```python
from build123d import *

# Parameters (mm, degrees)
BOSS_EXTRUDE1_DEPTH = 11
SHELL2_T            = -1.75
SKETCH5_W           = 10
SKETCH5_H           = 10.669048105
BOSS_EXTRUDE2_DEPTH = 9.25
HOLE4_D             = 4
HOLE4_DEPTH         = 13
HOLE4_CBORE_D       = 8
HOLE4_CBORE_DEPTH   = 5.5
HOLE4_TIP           = 1.201721238


with BuildPart() as part:
    # Sketch1 → Boss-Extrude1 (new body)
    with BuildSketch(Plane(origin=(0, 0, 0), x_dir=(1, 0, 0), z_dir=(0, 1, 0))):
        with BuildLine():
            Line((-12, -7.169048105), (-12, 13))
            Line((-12, 13), (12, 13))
            Line((12, 13), (12, -7.169048105))
            ThreePointArc((12, -7.169048105), (11.350863635, -11.062362212), (9.473684211, -14.534461025))
            ThreePointArc((9.473684211, -14.534461025), (7.719611593, -14.754072618), (7.5, -13))
            ThreePointArc((7.5, -13), (0, 2.330951895), (-7.5, -13))
            ThreePointArc((-7.5, -13), (-7.719611593, -14.754072618), (-9.473684211, -14.534461025))
            ThreePointArc((-9.473684211, -14.534461025), (-11.350863635, -11.062362212), (-12, -7.169048105))
        make_face()
    extrude(amount=BOSS_EXTRUDE1_DEPTH)

    # Shell2
    shell2_openings = [part.faces().sort_by_distance(p)[0] for p in [
        (0, 11, -3.682863913),
    ]]
    offset(amount=SHELL2_T, openings=shell2_openings, kind=Kind.INTERSECTION)

    # Sketch5 → Boss-Extrude2 (add)
    with BuildSketch(Plane(origin=(0, 11, 0), x_dir=(1, 0, 0), z_dir=(0, 1, 0))):
        with Locations((0, 7.665475948)):
            Rectangle(SKETCH5_W, SKETCH5_H)
    extrude(amount=-BOSS_EXTRUDE2_DEPTH)

    # Hole4
    with Locations(Plane.XY):
        with Locations((0, 5.5)):
            CounterBoreHole(HOLE4_D / 2, HOLE4_CBORE_D / 2, HOLE4_CBORE_DEPTH, depth=HOLE4_DEPTH)
            with Locations((0, 0, -(HOLE4_DEPTH + HOLE4_TIP / 2))):  # 118° drill point
                Cone(0, HOLE4_D / 2, HOLE4_TIP, mode=Mode.SUBTRACT)


solid = part.part
```
Build history of the part. All positions in model axes, mm. A direction names the side the tool comes from. Round coordinates to 2 decimals unless told otherwise and drop trailing zeros. Write each loop counter-clockwise with the first axis right and the second up, starting at its lowest first coordinate (ties: lowest second). Pieces come first, ordered by that corner, then holes.
1) Band-saw the part on B-B, the plane z = -6. List the corners of the cut face in (x, y).
2) Mould opens along Y. For faces 3 (the cylindrical face through (-7.7, 5.42, 14.74)), 4 (the cylindrical face through (2.15, 8.873, -3.446)), 5 (the flat face through (-8, 1.75, -6)) say: +Y half, -Y half, draft (parallel to the pull), parting line (faces both ways), or undercut.
3) 3-axis set-ups, long thin cutter, end or side, ignore diameter. For faces 1 (the flat face through (0, 3, -13)), 2 (the flat face through (5, 6, -7)): which of +Z, -Z, +X, -X, +Y, -Y reach the whole face in a straight line?
4) Band-saw the part on A-A, the plane y = 5.5. List the corners of the cut face in (x, z), and give its area (3 significant figures).
5) Pin check, flat tips, straight feed: pin 1 (4 mm diameter, centred on x = 6.5, y = 8.5, fed in from +Z); pin 2 (4 mm diameter, centred on x = -7.5, z = -5.5, fed in from +Y); pin 3 (2 mm diameter, centred on x = -0.5, y = 7.5, fed in from +Z); pin 4 (5 mm diameter, centred on x = 2.5, y = 1, fed in from +Z). Stop position of each tip, or through.
6) Band-saw the part on C-C, the plane x = 0. List the corners of the cut face in (y, z).
7) Band-saw the part on D-D, the plane z = 6.25. List the corners of the cut face in (x, y), and give its area (3 significant figures).
8) Drill centre lines: probe 1 along X at (y, z) = (5.5, -4.55); probe 2 along X at (y, z) = (9.75, 7); probe 3 along Y at (x, z) = (0, -8). Where is each one in solid material? Low to high.
Ans:
1. outline: (-12, 0) - (12, 0) - (12, 11) - (10.25, 11) - (10.25, 1.75) - (5, 1.75) - (5, 11) - (-5, 11) - (-5, 1.75) - (-10.25, 1.75) - (-10.25, 11) - (-12, 11) - close; hole circle Ø4 at (0, 5.5)
2. face 3: draft
2. face 4: undercut
2. face 5: +Y half
3. face 1: -Z, +X, -X, +Y, -Y
3. face 2: +Y
4. outline: (-12, -13) - (-2, -13) - (-2, -5.5) - (-4, -5.5) - (-4, -1.45) arc R9.5 cw to (-7.5, 13) arc R1.25 ccw to (-9.47, 14.53) arc R12 ccw to (-12, 7.17) - close; (2, -13) - (12, -13) - (12, 7.17) arc R12 ccw to (9.47, 14.53) arc R1.25 ccw to (7.5, 13) arc R9.5 cw to (4, -1.45) - (4, -5.5) - (2, -5.5) - close; hole (-10.25, -11.25) - (-5, -11.25) - (-5, -2.91) arc R11.25 cw to (-10.25, 2.53) - close; hole (5, -11.25) - (10.25, -11.25) - (10.25, 2.53) arc R11.25 cw to (5, -2.91) - close
4. area: 216 mm2
5. pin 1: stops at z = 15.02
5. pin 2: stops at y = 1.75
5. pin 3: stops at z = -5.5
5. pin 4: stops at z = -0.91
6. outline: (0, -13) - (3.5, -13) - (3.5, -5.5) - (1.5, -5.5) - (1.5, -2.33) - (0, -2.33) - close; (7.5, -13) - (11, -13) - (11, -2.33) - (9.5, -2.33) - (9.5, -5.5) - (7.5, -5.5) - close
7. outline: (-12, 0) - (-9.46, 0) - (-9.46, 11) - (-12, 11) - close; (9.46, 0) - (12, 0) - (12, 11) - (9.46, 11) - close
7. area: 56.0 mm2
8. probe 1: x = -12 to -10.25, -5 to -4, 4 to 5, 10.25 to 12
8. probe 2: x = -12 to -9.5, 9.5 to 12
8. probe 3: y = 0 to 3.5, 7.5 to 11
